Can you work these out from the model? Positions are in its coordinate system, mm. Coordinates: 2 decimals unless noted, no trailing zeros. Order: outer loops, then holes, each group sorted by start corner. A loop starts at its lowest first (then second) coordinate and runs counter-clockwise, first axis right, second up. Notation, with made-up numbers: (-37, 81.5) -> (-23, 81.5) arc R27 ccw to (-23, 104.5) -> close; hole circle Ø1 at (63, 19.25). An arc over 180 degrees is marked (long way). Use a Markdown table: item, result. Add a question column.
1. We'd pull the mould along Z, two halves only. Please class faces 1 (the cylindrical face through (-10.758, 0.493, 0.208)), 2 (the flat face through (-10.9, 0.5, 10.76)), 3 (the flat face through (-15, 0, 0)): pulls with the +Z half, pulls with the -Z half, needs draft (parallel to the pull), parting line crosses it, or undercut.
2. If I drill on line 1 along Z through (x, y) = (-4, 0.5); line 2 along Z through (x, y) = (-5.5, 0.65); line 3 along X through (y, z) = (0.3, -6.5), over which ranges is the centre line in solid material (lowest first)? Write a range as from..to.
3. Suppose I cut it at D-D, the plane z = -4.25. List the corners of the cut face in (x, y) for me.
4. Suppose I cut it at C-C, the plane x = -10.5. List the corners of the cut face in (y, z) for me.
5. Suppose I cut it at B-B, the plane x = -3.5. List the corners of the cut face in (y, z) for me.
```python
from build123d import *

# Parameters (mm, degrees)
BOSS_EXTRUDE1_DEPTH = 1
FILLET1_R           = 0.1
FILLET2_R           = 0.1
FILLET3_R           = 0.1
FILLET4_R           = 0.1


with BuildPart() as part:
    # Sketch1 → Boss-Extrude1 (new body)
    with BuildSketch(Plane(origin=(0, 0, 0), x_dir=(1, 0, 0), z_dir=(0, 1, 0))):
        with BuildLine():
            ThreePointArc((0, -10.76), (-10.76, 0), (0, 10.76))
            Line((0, 10.76), (-19.469525546, 10.76))
            ThreePointArc((-19.469525546, 10.76), (-22.245, 0), (-19.469525546, -10.76))
            Line((-19.469525546, -10.76), (0, -10.76))
        make_face()
    extrude(amount=BOSS_EXTRUDE1_DEPTH)

    # Fillet1
    fillet1_edges = [part.edges().sort_by_distance(p)[0] for p in [
        (0, 0.5, 10.76),
    ]]
    fillet(fillet1_edges, radius=FILLET1_R)

    # Fillet2
    fillet2_edges = [part.edges().sort_by_distance(p)[0] for p in [
        (0, 0.5, -10.76),
    ]]
    fillet(fillet2_edges, radius=FILLET2_R)

    # Fillet3
    fillet3_edges = [part.edges().sort_by_distance(p)[0] for p in [
        (-19.469525546, 0.5, 10.76),
    ]]
    fillet(fillet3_edges, radius=FILLET3_R)

    # Fillet4
    fillet4_edges = [part.edges().sort_by_distance(p)[0] for p in [
        (-19.469525546, 0.5, -10.76),
    ]]
    fillet(fillet4_edges, radius=FILLET4_R)


solid = part.part
```
Worked out:
| question | item | result |
|---|---|---|
| 1 | face 1 | undercut |
| 1 | face 2 | pulls with the +Z half |
| 1 | face 3 | needs draft |
| 2 | line 1 | z = -10.76..-9.99, 9.99..10.76 |
| 2 | line 2 | z = -10.76..-9.25, 9.25..10.76 |
| 2 | line 3 | x = -21.27..-8.57 |
| 3 | outline | (-21.84, 0) -> (-9.89, 0) -> (-9.89, 1) -> (-21.84, 1) -> close |
| 4 | outline | (0, -10.76) -> (1, -10.76) -> (1, -2.35) -> (0, -2.35) -> close; (0, 2.35) -> (1, 2.35) -> (1, 10.76) -> (0, 10.76) -> close |
| 5 | outline | (0, -10.76) -> (1, -10.76) -> (1, -10.17) -> (0, -10.17) -> close; (0, 10.17) -> (1, 10.17) -> (1, 10.76) -> (0, 10.76) -> close |
